Geometry check sheet. Reference: the model listing, model coordinates, mm. A direction names the side the tool comes from. Give positions to 0.01 mm unless a question says otherwise; leave off trailing zeros. Loops run counter-clockwise (first coordinate to the right, second up) from the corner with the lowest first, then second, coordinate; pieces in that order, holes last. Notation, with made-up numbers: (43.25, 42.25) - (76.25, 42.25) arc R30 cw to (76.25, 75.25) - close; hole circle Ø4 at (65, 25.5). An arc over 180 degrees is marked (long way). Use a Markdown table: item, result. Add a question column.
1. Cross-section at B-B on x = 25.5. Enter the section's corners in (y, z), and give its area (3 significant figures).
2. Depth check by flat-ended pin: P1, Ø17.5, axis at x = 54.5, y = 51, coming from the -Z side; P2, Ø11, axis at x = 35, z = -5, coming from the -Y side; P3, Ø3, axis at y = 13, z = -19.5, coming from the +X side. Enter the tip coordinate at first touch or a pass-through.
3. Cross-section at D-D on x = -11. Enter the section's corners in (y, z).
4. Draft check along X on faces 6 (the flat face through (23, 11, -12.5)), 7 (the flat face through (33.572, 13, 19)), 8 (the flat face through (-22, 35, -25)). Enter one of: pulls with the +X half, pulls with the -X half, needs draft (parallel to the pull), parting line crosses it, or undercut.
5. Set-up check for faces 1 (the flat face through (18.572, 0, 19)), 2 (the cylindrical face through (-42.907, 61.865, 0.35)), 3 (the flat face through (-46, 8, -12.5)), 4 (the flat face through (36, 42.578, 0)), 5 (the flat face through (25, 21.54, 0)): record each of +Z, -Z, +X, -X, +Y, -Y from which the full face is reachable in a straight line by a thin tool's end or side.
6. Material ranges on L1, parallel to Z at x = -52, y = 20; L2, parallel to X at y = 15.5, z = -21.5; L3, parallel to Y at x = 26, z = 19, recorded low to high.
7. Cross-section at A-A on z = 16.5. Enter the section's corners in (x, y) (1 decimal).
from build123d import *

# Parameters (mm, degrees)
F1_DEPTH     = 25
F2_DEPTH     = 12.5
F4_DEPTH     = 12.5
F5_DEPTH     = 16.25
F7_DEPTH     = 24.3842223705
F6_W         = 10
F6_H         = 10
F8_DEPTH     = 40
F10_DEPTH    = 20
F11_W        = 7.0710678119
F11_H        = 20
F12_ANGLE    = 180
F13_W        = 25
F13_H        = 50
F13_W_2      = 11.2650044263
F14_ANGLE    = 5.7295779513
F15_T1_DEPTH = 52.2024679969
F15_T3_DEPTH = 69.535784442
F15_T6_ANGLE = 45.7032352823
F15_T8_ANGLE = 45.7032352823


# Not quite as in the source:
# - a fillet or chamfer that OpenCascade refuses, or shapes differently, is made with other operations: its cross-section is extruded or revolved along the edge and cut away or added
# - a pattern or mirror of a feature is missing from the dataset's text; its kind, count and spacing are read off the source's solid


with BuildPart() as f1:
    # F0 (on Top) → F1 (new body)
    with BuildSketch(Plane.XY):
        with BuildLine():
            ThreePointArc((8.5724992678, 52.5779476486), (-17.4169661561, 54.4628096646), (-42.8625009954, 60.0779476486))
            Line((-42.8625009954, 60.0779476486), (-79.1275054216, 60.0779476486))
            ThreePointArc((-79.1275054216, 60.0779476486), (-73.2024272044, 46.6744306132), (-71.1757168174, 32.1605315572))
            ThreePointArc((-71.1757168174, 32.1605315572), (-67.4004664777, 26.1656086442), (-60.7126449392, 23.8279476486))
            ThreePointArc((-60.7126449392, 23.8279476486), (-57.8761392565, 22.6699366601), (-56.2426317111, 20.0779476486))
            Line((-56.2426317111, 20.0779476486), (-56.2426317111, 27.5779476486))
            Line((-56.2426317111, 27.5779476486), (-42.8625009954, 27.5779476486))
            ThreePointArc((-42.8625009954, 27.5779476486), (-39.3668172692, 25.5518582213), (-35.7126449392, 23.8279476486))
            ThreePointArc((-35.7126449392, 23.8279476486), (-14.2067307678, 20.1682602333), (6.6882768972, 26.4369372072))
            ThreePointArc((6.6882768972, 26.4369372072), (11.5749679763, 31.8294833583), (18.5724992678, 33.8279476486))
            Line((18.5724992678, 33.8279476486), (18.5724992678, 40.0779476486))
            Line((18.5724992678, 40.0779476486), (18.5724992678, 52.5779476486))
            Line((18.5724992678, 52.5779476486), (8.5724992678, 52.5779476486))
        make_face()
        with BuildLine():
            Line((-56.2426317111, 27.5779476486), (-56.2426317111, 20.0779476486))
            ThreePointArc((-56.2426317111, 20.0779476486), (-56.084348871, 18.8279476486), (-56.2426317111, 17.5779476486))
            Line((-56.2426317111, 17.5779476486), (-52.8975990321, -12.4220523514))
            Line((-52.8975990321, -12.4220523514), (-39.2875729673, -12.4220523514))
            Line((-39.2875729673, -12.4220523514), (-35.7126449392, 23.8279476486))
            ThreePointArc((-35.7126449392, 23.8279476486), (-39.3668172692, 25.5518582213), (-42.8625009954, 27.5779476486))
            Line((-42.8625009954, 27.5779476486), (-56.2426317111, 27.5779476486))
        make_face()
        with BuildLine():
            ThreePointArc((29.8224992678, 27.5779476486), (25.0072681059, 32.1605315572), (18.5724992678, 33.8279476486))
            ThreePointArc((18.5724992678, 33.8279476486), (11.5749679763, 31.8294833583), (6.6882768972, 26.4369372072))
            ThreePointArc((6.6882768972, 26.4369372072), (10.35454594, 17.5558849939), (18.5724992678, 12.5779476486))
            Line((18.5724992678, 12.5779476486), (18.5724992678, -12.4220523514))
            Line((18.5724992678, -12.4220523514), (29.8224992678, -12.4220523514))
            Line((29.8224992678, -12.4220523514), (33.5724992678, 7.5779476486))
            Line((33.5724992678, 7.5779476486), (33.5724992678, 17.5779476486))
            ThreePointArc((33.5724992678, 17.5779476486), (30.7908263589, 22.2379453078), (29.8224992678, 27.5779476486))
        make_face()
    extrude(amount=F1_DEPTH)

    # F0 (on Top) → F2 (cut)
    with BuildSketch(Plane.XY):
        with BuildLine():
            ThreePointArc((29.8224992678, 27.5779476486), (25.0072681059, 32.1605315572), (18.5724992678, 33.8279476486))
            ThreePointArc((18.5724992678, 33.8279476486), (11.5749679763, 31.8294833583), (6.6882768972, 26.4369372072))
            ThreePointArc((6.6882768972, 26.4369372072), (10.35454594, 17.5558849939), (18.5724992678, 12.5779476486))
            Line((18.5724992678, 12.5779476486), (18.5724992678, -12.4220523514))
            Line((18.5724992678, -12.4220523514), (29.8224992678, -12.4220523514))
            Line((29.8224992678, -12.4220523514), (33.5724992678, 7.5779476486))
            Line((33.5724992678, 7.5779476486), (33.5724992678, 17.5779476486))
            ThreePointArc((33.5724992678, 17.5779476486), (30.7908263589, 22.2379453078), (29.8224992678, 27.5779476486))
        make_face()
        with BuildLine():
            Line((-56.2426317111, 27.5779476486), (-56.2426317111, 20.0779476486))
            ThreePointArc((-56.2426317111, 20.0779476486), (-56.084348871, 18.8279476486), (-56.2426317111, 17.5779476486))
            Line((-56.2426317111, 17.5779476486), (-52.8975990321, -12.4220523514))
            Line((-52.8975990321, -12.4220523514), (-39.2875729673, -12.4220523514))
            Line((-39.2875729673, -12.4220523514), (-35.7126449392, 23.8279476486))
            ThreePointArc((-35.7126449392, 23.8279476486), (-39.3668172692, 25.5518582213), (-42.8625009954, 27.5779476486))
            Line((-42.8625009954, 27.5779476486), (-56.2426317111, 27.5779476486))
        make_face()
    extrude(amount=F2_DEPTH, mode=Mode.SUBTRACT)

    # F3: F1 across plane


with BuildPart() as f1_1:
    add(f1.part)
    add(f1.part.mirror(Plane.XY))

    # F4 (add): a face of the model
    f4_faces = [f1_1.faces().sort_by_distance(p)[0] for p in [
        (18.5724992678, 43.2029476486, 0),
    ]]
    extrude(f4_faces, amount=F4_DEPTH)

    # F5 (add, through all): a face of the model
    f5_faces = [f1_1.faces().sort_by_distance(p)[0] for p in [
        (24.8224992678, 33.8279476486, 0),
    ]]
    extrude(f5_faces, amount=F5_DEPTH)

    # F6 (on face) → F7 (cut, through all)
    with BuildSketch(Plane.YZ.offset(31.0724992678)):
        Polygon((21.5398740044, 0), (21.5398740044, 12.5), (17.5779476486, 12.5), (17.5779476486, -12.5), (21.5398740044, -12.5), align=None)
    extrude(amount=-F7_DEPTH, mode=Mode.SUBTRACT)

    # F6 (on face) → F8 (join)
    with BuildSketch(Plane.YZ.offset(31.0724992678)):
        Polygon((62.5779476486, 10), (52.5779476486, 10), (52.5779476486, 0), (52.5779476486, -10), (62.5779476486, -10), align=None)
        with Locations((47.5779476486, 5)):
            Rectangle(F6_W, F6_H)
    f8 = extrude(amount=F8_DEPTH)

    # F8_copies: F8 across plane
    add(f8.mirror(Plane(origin=(0, 0, 0), x_dir=(-1, 0, 0), z_dir=(0, 0, -1))))

    # F9 (on face) → F10 (cut, through all)
    with BuildSketch(Plane.XY.offset(10)):
        with BuildLine():
            ThreePointArc((31.0724992678, 52.5779476486), (46.8838875686, 55.1437827461), (61.0724992678, 62.5779476486))
            Line((61.0724992678, 62.5779476486), (51.0724992678, 62.5779476486))
            Line((51.0724992678, 62.5779476486), (31.0724992678, 62.5779476486))
            Line((31.0724992678, 62.5779476486), (31.0724992678, 52.5779476486))
        make_face()
        Polygon((71.0724992678, 52.5779476486), (71.0724992678, 62.5779476486), (61.0724992678, 62.5779476486), align=None)
        with BuildLine():
            Line((71.0724992678, 42.5779476486), (71.0724992678, 52.5779476486))
            ThreePointArc((71.0724992678, 52.5779476486), (55.2611109669, 50.0121125511), (41.0724992678, 42.5779476486))
            Line((41.0724992678, 42.5779476486), (51.0724992678, 42.5779476486))
            Line((51.0724992678, 42.5779476486), (71.0724992678, 42.5779476486))
        make_face()
    extrude(amount=-F10_DEPTH, mode=Mode.SUBTRACT)

    # F11 (on face) → F12 (revolve)
    with BuildSketch(Plane(origin=(61.8252234582, 61.8252234582, 0), x_dir=(-0.7071067812, 0.7071067812, 0), z_dir=(0.7071067812, 0.7071067812, 0))):
        with Locations((-2.4710211471, 0)):
            Rectangle(F11_W, F11_H)
    revolve(axis=Axis((66.0724992678, 57.5779476486, 0), (0, 0, -1)), revolution_arc=F12_ANGLE)

    # F13 (on face) → F14 (revolve)
    with BuildSketch(Plane(origin=(0, 60.0779476486, 0), x_dir=(-1, 0, 0), z_dir=(0, 1, 0))):
        with Locations((55.3625009954, 0)):
            Rectangle(F13_W, F13_H)
        with Locations((73.4950032085, 0)):
            Rectangle(F13_W_2, F13_H)
    revolve(axis=Axis((-79.1275054216, 60.0779476486, 0), (0, 0, 1)), revolution_arc=F14_ANGLE)

    # F15: chamfer of 2.5 on 4 edges, made by hand

    # F15_s2 → F15_t1 (cut)
    with BuildSketch(Plane.XY.offset(-26.1012339984)):
        with BuildLine():
            Line((-71.1765205144, 32.4523590493), (-71.0941336441, 31.829473599))
            ThreePointArc((-71.0941336441, 31.829473599), (-71.1242415299, 31.9464717064), (-71.1757168174, 32.1605315572))
            ThreePointArc((-71.1757168174, 32.1605315572), (-71.1760775289, 32.3560379433), (-71.1765205144, 32.4523590493))
        make_face()
    extrude(amount=F15_T1_DEPTH, mode=Mode.SUBTRACT)

    # F15_s4 → F15_t3 (cut)
    with BuildSketch(Plane.XY.offset(-34.767892221)):
        with BuildLine():
            Line((-77.2597253727, 56.8116607658), (-75.2963846316, 60.4623418968))
            Line((-75.2963846316, 60.4623418968), (-79.1275054216, 60.0779476486))
            ThreePointArc((-79.1275054216, 60.0779476486), (-78.1514580859, 58.4383743549), (-77.2597253727, 56.8116607658))
        make_face()
    extrude(amount=F15_T3_DEPTH, mode=Mode.SUBTRACT)

    # F15_s5 → F15_t6 (revolve, cut)
    with BuildSketch(Plane(origin=(-64.3425340859, 80.1682893814, 0), x_dir=(0, 0, 1), z_dir=(-0.6259274923, 0.7798812566, 0))):
        Polygon((22.5, -23.7159805894), (25, -21.2159805894), (25, -23.7159805894), align=None)
    revolve(axis=Axis((-124.1583289793, 32.1605315572, 25), (0, 0, -1)), revolution_arc=F15_T6_ANGLE, mode=Mode.SUBTRACT)

    # F15_s7 → F15_t8 (revolve, cut)
    with BuildSketch(Plane(origin=(-64.3425340859, 80.1682893814, 0), x_dir=(0, 0, 1), z_dir=(-0.6259274923, 0.7798812566, 0))):
        Polygon((-25, -21.2159805894), (-22.5, -23.7159805894), (-25, -23.7159805894), align=None)
    revolve(axis=Axis((-124.1583289793, 32.1605315572, -25), (0, 0, -1)), revolution_arc=F15_T8_ANGLE, mode=Mode.SUBTRACT)


solid = f1_1.part
Values found:
| question | item | result |
|---|---|---|
| 1 | outline | (-12.42, -25) - (52.58, -25) - (52.58, 25) - (-12.42, 25) - (-12.42, 12.5) - (21.54, 12.5) - (21.54, -12.5) - (-12.42, -12.5) - close |
| 1 | area | 2,400 mm2 |
| 2 | P1 | stops at z = -10 |
| 2 | P2 | stops at y = 21.54 |
| 2 | P3 | stops at x = 33.57 |
| 3 | outline | (20.47, -25) - (53.64, -25) - (53.64, 25) - (20.47, 25) - close |
| 4 | face 6 | undercut |
| 4 | face 7 | pulls with the +X half |
| 4 | face 8 | needs draft |
| 5 | face 1 | +Z, -Z, -Y |
| 5 | face 2 | +Z, -Z, +Y |
| 5 | face 3 | -Y |
| 5 | face 4 | +Z, -Z, +X, -Y |
| 5 | face 5 | +X, -Y |
| 6 | L1 | z = -25 to -12.5, 12.5 to 25 |
| 6 | L2 | x = -56.01 to -36.53, 12.49 to 33.57 |
| 6 | L3 | y = -12.42 to 52.58 |
| 7 | outline | (-77.3, 56.8) arc R53 cw to (-71.2, 32.5) - (-71.1, 31.8) arc R10.7 ccw to (-60.7, 23.8) arc R5 cw to (-56.2, 17.6) - (-52.9, -12.4) - (-39.3, -12.4) - (-35.7, 23.8) arc R47.8 ccw to (6.7, 26.4) arc R15.4 ccw to (18.6, 12.6) - (18.6, -12.4) - (29.8, -12.4) - (33.6, 7.6) - (33.6, 17.6) arc R15.2 cw to (31.1, 21.5) - (31.1, 52.6) - (8.6, 52.6) arc R180.1 cw to (-42.9, 60.1) arc R36.3 ccw to (-43, 63.7) - (-75.3, 60.5) - close |
